Build history of the part. All positions in model axes, mm. A direction names the side the tool comes from. Round coordinates to 2 decimals unless told otherwise and drop trailing zeros. Loops run counter-clockwise (first coordinate to the right, second up) from the corner with the lowest first, then second, coordinate; pieces in that order, holes last. Notation, with made-up numbers: (-10.75, 54.25) - (46.25, 54.25) arc R23 ccw to (46.25, 63.25) - close; hole circle Ø4 at (-20, 65). An arc over 180 degrees is marked (long way). Use a Markdown table: item, result.
from build123d import *

# Parameters (mm, degrees)
SKETCH_1_R          = 3
EXTRUDE_1_DEPTH     = 21.05
SKETCH_2_R          = 1.5
EXTRUDE_2_DEPTH     = 1
SKETCH_3_R          = 1
EXTRUDE_3_DEPTH     = 2.6
CUT_EXTRUDE_1_DEPTH = 2.5
FILLET_1_R          = 0.25


with BuildPart() as part:
    # 草图1 → 凸台-拉伸1 (new body)
    with BuildSketch(Plane.XY):
        Circle(SKETCH_1_R)
    extrude(amount=-EXTRUDE_1_DEPTH)

    # 草图2 → 凸台-拉伸2 (add)
    with BuildSketch(Plane.XY):
        Circle(SKETCH_2_R)
    extrude(amount=EXTRUDE_2_DEPTH)

    # 草图3 → 凸台-拉伸3 (add)
    with BuildSketch(Plane.XY.offset(1)):
        Circle(SKETCH_3_R)
    extrude(amount=EXTRUDE_3_DEPTH)

    # 草图4 → 切除-拉伸1 (cut)
    with BuildSketch(Plane.XY.offset(3.6)):
        Polygon((0, -0.5), (0.862464595, -0.5), (0.862464595, -1), (0, -1), (-0.86936686, -1), (-0.86936686, -0.5), align=None)
    extrude(amount=-CUT_EXTRUDE_1_DEPTH, mode=Mode.SUBTRACT)

    # 圆角1
    fillet_1_edges = [part.edges().sort_by_distance(p)[0] for p in [
        (-1.5, 0, 1),
    ]]
    fillet(fillet_1_edges, radius=FILLET_1_R)


solid = part.part
Q1. Cut at D-D, the plane z = 0.25. List the corners of the cut face in (x, y), plus the area to 3 significant figures.
Results found:
| item | result |
|---|---|
| outline | circle Ø3 at (0, 0) |
| area | 7.07 mm2 |
Q2. Cut at C-C, the plane z = -13.75. List the corners of the cut face in (x, y), plus the area to 3 significant figures.
Results found:
| item | result |
|---|---|
| outline | circle Ø6 at (0, 0) |
| area | 28.3 mm2 |
Q3. Cut at B-B, the plane x = 0. List the corners of the cut face in (y, z).
Results found:
| item | result |
|---|---|
| outline | (-3, -21.05) - (3, -21.05) - (3, 0) - (1.5, 0) - (1.5, 0.75) arc R0.25 ccw to (1.25, 1) - (1, 1) - (1, 3.6) - (-0.5, 3.6) - (-0.5, 1.1) - (-1, 1.1) - (-1, 1) - (-1.25, 1) arc R0.25 ccw to (-1.5, 0.75) - (-1.5, 0) - (-3, 0) - close |
Q4. Cut at A-A, the plane y = 0. List the corners of the cut face in (x, z), plus the area to 3 significant figures.
Results found:
| item | result |
|---|---|
| outline | (-3, -21.05) - (3, -21.05) - (3, 0) - (1.5, 0) - (1.5, 0.75) arc R0.25 ccw to (1.25, 1) - (1, 1) - (1, 3.6) - (-1, 3.6) - (-1, 1) - (-1.25, 1) arc R0.25 ccw to (-1.5, 0.75) - (-1.5, 0) - (-3, 0) - close |
| area | 134 mm2 |
Q5. Drop flat-ended pins along their axis: pin 1 (0.9 mm diameter, centred on x = 0, z = 2, fed in from -Y); pin 2 (1 mm diameter, centred on x = -2.5, y = 0.5, fed in from +Z). Give the stop position or say it passes through.
Results found:
| item | result |
|---|---|
| pin 1 | stops at y = -0.5 |
| pin 2 | stops at z = 0 |
Q6. Probe line 1 (X direction, y = 2.6, z = -5.75); line 2 (Z direction, x = -1.65, y = -2.15); line 3 (Y direction, x = 0.1, z = 1.75). List the from-to ranges inside material, lowest first.
Results found:
| item | result |
|---|---|
| line 1 | x = -1.5 to 1.5 |
| line 2 | z = -21.05 to 0 |
| line 3 | y = -0.5 to 0.99 |
Q7. Which spindle directions (+Z, -Z, +X, -X, +Y, -Y) get a long thin tool onto all of the face, cutting with end or side? Do faces 1 (the face through (1.3, -1.3, 0)), 2 (the face through (-3, 0, -10)). Say none if no direction does.
Results found:
| item | result |
|---|---|
| face 1 | +Z |
| face 2 | +Z, -Z |
